Autodesk Inventor part; units mm, degrees
ref_plane "YZ Plane" through (0, 0, 0) normal (1, 0, 0) x (0, 1, 0)
ref_plane "XZ Plane" through (0, 0, 0) normal (0, 1, 0) x (-1, 0, 0)
ref_plane "XY Plane" through (0, 0, 0) normal (0, 0, 1) x (1, 0, 0)
sketch "Sketch1" plane through (0, 0, 0) normal (0, 1, 0) x (-1, 0, 0)
  line L0 (0, 0) -> (150, 0)
  line L1 (150, 0) -> (150, -200)
  line L2 (150, -200) -> (0, -200)
  line L3 (0, -200) -> (0, 0)
  line L4 (150, -200) -> (150, -143.8709)
  dimension "d0" = 150
  dimension "d1" = 200
extrude "Extrusion1" add sketch "Sketch1" along normal blind 10
sketch "Sketch3" plane through (0, 0, 0) normal (0, -1, 0) x (1, 0, 0)
  line L0 (-85, -199.8) -> (-85, -213.2303) construction
  line L1 (0, -200) -> (-150, -200)
  line L2 (-75, -213.1946) -> (-89.7696, -213.1946)
  arc A0 (-90.4946, -212.0565) -> (-89.7696, -213.1946) centre (-89.7696, -212.3946) ccw
  line L3 (-90.4946, -212.0565) -> (-84.8726, -200)
  line L4 (-84.8726, -200) -> (-65.1274, -200)
  line L5 (-65.1274, -200) -> (-59.5054, -212.0565)
  arc A1 (-60.2304, -213.1946) -> (-59.5054, -212.0565) centre (-60.2304, -212.3946) ccw
  line L6 (-60.2304, -213.1946) -> (-75, -213.1946)
  line L7 (-149.8, -90) -> (-163.2303, -90) construction
  line L8 (-163.1946, -100) -> (-163.1946, -85.2304)
  arc A2 (-162.0565, -84.5054) -> (-163.1946, -85.2304) centre (-162.3946, -85.2304) ccw
  line L9 (-162.0565, -84.5054) -> (-150, -90.1274)
  line L10 (-150, -90.1274) -> (-150, -109.8726)
  line L11 (-150, -109.8726) -> (-162.0565, -115.4946)
  arc A3 (-163.1946, -114.7696) -> (-162.0565, -115.4946) centre (-162.3946, -114.7696) ccw
  line L12 (-163.1946, -114.7696) -> (-163.1946, -100)
  line L13 (-150, -200) -> (-150, 0)
  point P0 (0, 0)
  point P1 (-75, -200)
  point P2 (-75, -200)
  point P3 (-150, -100)
  point P4 (-150, -100)
  point P5 (-150, -100)
extrude "Extrusion3" add sketch "Sketch3" against normal blind 4.8
sketch "Sketch5" plane through (0, 10, 0) normal (0, 1, 0) x (1, 0, 0)
  line L0 (-150, 200) -> (-150, 0)
  line L1 (-150, 0) -> (-75, 0)
  line L2 (-150, 0) -> (0, 0)
  line L3 (-75, 0) -> (-75, 75)
  circle A0 centre (-75, 75) radius 2.5
  circle A1 centre (-75, 75) radius 2.6
  line L4 (-150, 200) -> (-150, 0)
  line L5 (-150, 200) -> (-75, 200)
  line L6 (0, 200) -> (-150, 200)
  circle A2 centre (-75, 200) radius 2.5
  circle A3 centre (-75, 200) radius 2.6
  point P0 (-150, 89.7793)
  point P1 (-150, 110.2207)
  dimension "d17" = 75
  dimension "d18" = 5
  dimension "d19" = 0.1
  dimension "d20" = 5
  dimension "d21" = 0.1
extrude "Extrusion4" cut sketch "Sketch5" against normal blind 5.2 contours A0 | A1 | A3 L6 A2 L5 | L5 A2 L6 A3 | A2 L6 L5 | L5 L6 A2
sketch "Sketch7" plane through (0, 10, 0) normal (0, 1, 0) x (1, 0, 0)
  line L0 (0, 0) -> (0, 200)
  line L1 (-150, 0) -> (0, 0)
  line L2 (0, 200) -> (-50, 200)
  line L3 (-50, 200) -> (-50, 0)
  line L4 (-50, 0) -> (0, 0)
  line L5 (0, 0) -> (0, 200)
  line L6 (-150, 0) -> (0, 0)
  line L7 (0, 0) -> (0, 50)
  line L8 (0, 50) -> (-150, 50)
  line L9 (-150, 50) -> (-150, 0)
  line L10 (-150, 200) -> (-100, 200)
  line L11 (-100, 200) -> (-100, 130)
  line L12 (-100, 130) -> (-150, 130)
  line L13 (-150, 130) -> (-150, 200)
  point P0 (-50, 50)
  dimension "d24" = 50
  dimension "d25" = 50
  dimension "d26" = 50
  dimension "d27" = 70
extrude "Extrusion5" cut sketch "Sketch7" against normal blind 10
fillet "Fillet1" radius 10 6 edges at (-50, 5, -200) (-100, 5, -200) (-150, 5, -130) (-100, 5, -130) (-50, 5, -50) (-150, 5, -50)
properties part number "Area nv"
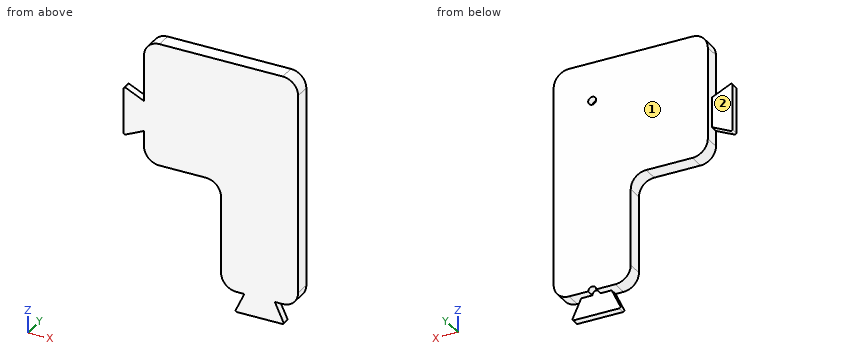
Model file for the job. Use its own axes, mm. Face numbers are marked on the shaded views. A direction names the side the tool comes from. Coordinates: 2 decimals unless noted, no trailing zeros. Loops run counter-clockwise (first coordinate to the right, second up) from the corner with the lowest first, then second, coordinate; pieces in that order, holes last. Notation, with made-up numbers: (-32, -1) -> (-7, -1) arc R17 cw to (-7, 4) -> close; hole circle Ø3 at (7.5, -37.5). An arc over 180 degrees is marked (long way). Answer as a JSON object with one key per item and string values.
Q1. Cut at A-A (y = 8.25). List the corners of the cut face in (x, z).
Report:
{"outline": "(-150, -120) arc R10 ccw to (-140, -130) -> (-110, -130) arc R10 cw to (-100, -140) -> (-100, -190) arc R10 ccw to (-90, -200) -> (-77.6, -200) arc R2.6 cw to (-72.4, -200) -> (-60, -200) arc R10 ccw to (-50, -190) -> (-50, -60) arc R10 ccw to (-60, -50) -> (-140, -50) arc R10 ccw to (-150, -60) -> close; hole circle Ø5.2 at (-75, -75)"}
Q2. Flat gauge pins, fed straight in: P1, Ø5, axis at x = -121.5, y = 7.5, coming from the -Z side; P2, Ø8, axis at x = -75.5, z = -203.5, coming from the +Y side; P3, Ø3, axis at y = 4, z = -172, coming from the -X side. Where does each tip first touch, or does it go through?
Report:
{"P1": "stops at z = -130", "P2": "stops at y = 4.8", "P3": "stops at x = -100"}
Q3. 3-axis set-ups, long thin cutter, end or side, ignore diameter. For the marked faces 1 and 2: which of +Z, -Z, +X, -X, +Y, -Y reach the whole face in a straight line?
Report:
{"face 1": "+Z, -Z, +X, -X, +Y", "face 2": "+Z, -Z, -X, +Y"}
Q4. Cut at D-D (z = -98). List the corners of the cut face in (x, y).
Report:
{"outline": "(-163.19, 0) -> (-50, 0) -> (-50, 10) -> (-150, 10) -> (-150, 4.8) -> (-163.19, 4.8) -> close"}
Q5. Cut at B-B (x = -75). List the corners of the cut face in (y, z), and give its area (3 significant figures).
Report:
{"outline": "(0, -213.19) -> (4.8, -213.19) -> (4.8, -197.4) -> (10, -197.4) -> (10, -77.6) -> (4.8, -77.6) -> (4.8, -72.4) -> (10, -72.4) -> (10, -50) -> (0, -50) -> close", "area": "1,520 mm2"}
Q6. Probe probe 1 along X at (y, z) = (7.35, -75); probe 2 along Z at (x, y) = (-75, 8.95); probe 3 along X at (y, z) = (1, -146). List the from-to ranges inside material, lowest first.
Report:
{"probe 1": "x = -150 to -77.6, -72.4 to -50", "probe 2": "z = -197.4 to -77.6, -72.4 to -50", "probe 3": "x = -100 to -50"}
Q7. Cut at C-C (z = -75). List the corners of the cut face in (x, y).
Report:
{"outline": "(-150, 0) -> (-50, 0) -> (-50, 10) -> (-72.4, 10) -> (-72.4, 4.8) -> (-77.6, 4.8) -> (-77.6, 10) -> (-150, 10) -> close"}
